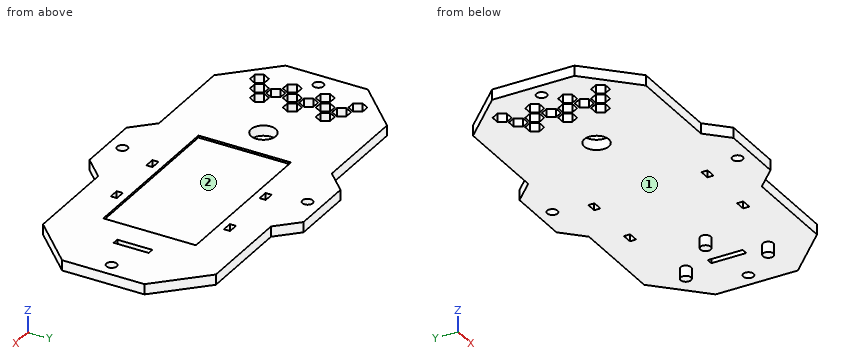
```python
from build123d import *

# Parameters (mm, degrees)
BASE_FLANGE1_OUTLINE_R  = 6
BASE_FLANGE1_DEPTH      = 5
SKETCH3_W               = 80
SKETCH3_H               = 45
CUT_EXTRUDE1_DEPTH      = 1
CROQUIS1_W              = 5
CROQUIS1_H              = 3
CORTAR_EXTRUIR1_DEPTH   = 108.540687679
CROQUIS2_R              = 2.5
CORTAR_EXTRUIR2_DEPTH   = 108.540687679
CROQUIS3_R              = 2.5
SALIENTE_EXTRUIR1_DEPTH = 5
CUT_EXTRUDE3_DEPTH      = 10
SKETCH9_W               = 3
SKETCH9_H               = 17
CUT_EXTRUDE4_DEPTH      = 10


# Read off the part's stored shape, not the designer's step: Base-Flange1
with BuildPart() as part:
    # Base-Flange1 outline → Base-Flange1 (new body)
    with BuildSketch(Plane(origin=(0, 0, 12.500000186), x_dir=(-1, 0, 0), z_dir=(0, 0, -1))):
        Polygon((-93.999996781, 19.999999553), (-93.999996781, -19.999999553), (-71.999996901, -41.999999434), (-25.556499138, -41.999999434), (-15.556500293, -52.000001073), (15.556500293, -52.000001073), (25.556499138, -41.999999434), (71.999996901, -41.999999434), (93.999996781, -19.999999553), (93.999996781, 19.999999553), (71.999996901, 41.999999434), (25.556499138, 41.999999434), (15.556500293, 52.000001073), (-15.556500293, 52.000001073), (-25.556499138, 41.999999434), (-71.999996901, 41.999999434), align=None)
        with Locations((40.791069868, 0)):
            Circle(BASE_FLANGE1_OUTLINE_R, mode=Mode.SUBTRACT)
    extrude(amount=BASE_FLANGE1_DEPTH)

    # Sketch3 → Cut-Extrude1 (cut)
    with BuildSketch(Plane.XY.offset(12.500000186)):
        with Locations((15, 0)):
            Rectangle(SKETCH3_W, SKETCH3_H)
    extrude(amount=-CUT_EXTRUDE1_DEPTH, mode=Mode.SUBTRACT)

    # Croquis1 → Cortar-Extruir1 (cut, through all)
    with BuildSketch(Plane.XY.offset(12.500000186)):
        with Locations((5, 27.5)):
            Rectangle(CROQUIS1_W, CROQUIS1_H)
        with Locations((35, 27.5)):
            Rectangle(CROQUIS1_W, CROQUIS1_H)
        with Locations((35, -27.5)):
            Rectangle(CROQUIS1_W, CROQUIS1_H)
        with Locations((5, -27.5)):
            Rectangle(CROQUIS1_W, CROQUIS1_H)
    extrude(amount=-CORTAR_EXTRUIR1_DEPTH, mode=Mode.SUBTRACT)

    # Croquis2 → Cortar-Extruir2 (cut, through all)
    with BuildSketch(Plane(origin=(0, 0, 7.500000186), x_dir=(-1, 0, 0), z_dir=(0, 0, -1))):
        with Locations((-86.999996781, 0)):
            Circle(CROQUIS2_R)
        with Locations(Location((86.999996781, 0, 0), (0, 0, 180))):
            Circle(CROQUIS2_R)
        with Locations((0, 45.000001073)):
            Circle(CROQUIS2_R)
        with Locations(Location((0, -45.000001073, 0), (0, 0, 180))):
            Circle(CROQUIS2_R)
    extrude(amount=-CORTAR_EXTRUIR2_DEPTH, mode=Mode.SUBTRACT)

    # Croquis3 → Saliente-Extruir1 (add)
    with BuildSketch(Plane(origin=(0, 0, 7.500000186), x_dir=(-1, 0, 0), z_dir=(0, 0, -1))):
        with Locations((-50.999996781, 0)):
            Circle(CROQUIS3_R)
        with Locations((-68.999996781, 20)):
            Circle(CROQUIS3_R)
        with Locations((-68.999996781, -20)):
            Circle(CROQUIS3_R)
    extrude(amount=SALIENTE_EXTRUIR1_DEPTH)

    # Sketch8 → Cut-Extrude3 (cut)
    with BuildSketch(Plane.XY.offset(12.500000186)):
        Polygon((-67.999996901, -19.999999553), (-69.999996901, -16.535897938), (-73.999996901, -16.535897938), (-75.999996901, -19.999999553), (-73.999996901, -23.464101168), (-69.999996901, -23.464101168), align=None)
        Polygon((-69.999996901, -8.607694708), (-67.999996901, -12.071796323), (-69.999996901, -15.535897938), (-73.999996901, -15.535897938), (-75.999996901, -12.071796323), (-73.999996901, -8.607694708), align=None)
        Polygon((-63.133971497, -19.499999553), (-67.133971497, -19.499999553), (-69.133971497, -16.035897938), (-67.133971497, -12.571796323), (-63.133971497, -12.571796323), (-61.133971497, -16.035897938), align=None)
        Polygon((-67.999996901, -3.999999553), (-69.999996901, -0.535897938), (-73.999996901, -0.535897938), (-75.999996901, -3.999999553), (-73.999996901, -7.464101168), (-69.999996901, -7.464101168), align=None)
        Polygon((-76.866022304, -27.428202783), (-80.866022304, -27.428202783), (-82.866022304, -23.964101168), (-80.866022304, -20.499999553), (-76.866022304, -20.499999553), (-74.866022304, -23.964101168), align=None)
        Polygon((-69.999996901, 7.392305292), (-67.999996901, 3.928203677), (-69.999996901, 0.464102062), (-73.999996901, 0.464102062), (-75.999996901, 3.928203677), (-73.999996901, 7.392305292), align=None)
        Polygon((-63.133971497, -3.499999553), (-67.133971497, -3.499999553), (-69.133971497, -0.035897938), (-67.133971497, 3.428203677), (-63.133971497, 3.428203677), (-61.133971497, -0.035897938), align=None)
        Polygon((-76.866022304, -11.428202783), (-80.866022304, -11.428202783), (-82.866022304, -7.964101168), (-80.866022304, -4.499999553), (-76.866022304, -4.499999553), (-74.866022304, -7.964101168), align=None)
        Polygon((-67.999996901, 12.000000447), (-69.999996901, 15.464102062), (-73.999996901, 15.464102062), (-75.999996901, 12.000000447), (-73.999996901, 8.535898832), (-69.999996901, 8.535898832), align=None)
        Polygon((-69.999996901, 23.392305292), (-67.999996901, 19.928203677), (-69.999996901, 16.464102062), (-73.999996901, 16.464102062), (-75.999996901, 19.928203677), (-73.999996901, 23.392305292), align=None)
        Polygon((-63.133971497, 12.500000447), (-67.133971497, 12.500000447), (-69.133971497, 15.964102062), (-67.133971497, 19.428203677), (-63.133971497, 19.428203677), (-61.133971497, 15.964102062), align=None)
        Polygon((-76.866022304, 4.571797217), (-80.866022304, 4.571797217), (-82.866022304, 8.035898832), (-80.866022304, 11.500000447), (-76.866022304, 11.500000447), (-74.866022304, 8.035898832), align=None)
        Polygon((-74.866022304, 23.892305292), (-76.866022304, 27.356406908), (-80.866022304, 27.356406908), (-82.866022304, 23.892305292), (-80.866022304, 20.428203677), (-76.866022304, 20.428203677), align=None)
    extrude(amount=-CUT_EXTRUDE3_DEPTH, mode=Mode.SUBTRACT)

    # Sketch9 → Cut-Extrude4 (cut)
    with BuildSketch(Plane.XY.offset(12.500000186)):
        with Locations((68.999996781, 0)):
            Rectangle(SKETCH9_W, SKETCH9_H)
    extrude(amount=-CUT_EXTRUDE4_DEPTH, mode=Mode.SUBTRACT)


solid = part.part
```
Here's how the part is built. I have some questions about the finished solid (model axes, mm). Face numbers are marked on the shaded views. Give positions to 0.01 mm unless a question says otherwise; leave off trailing zeros. Loops run counter-clockwise (first coordinate to the right, second up) from the corner with the lowest first, then second, coordinate; pieces in that order, holes last. Notation, with made-up numbers: M 58.5,86 L 64.5,86 A25 ccw 64.5,102 Z; hole C -14,47.25 d10. An arc over 180 degrees is marked long. Use one line per item in the form item = value. Start each with the question number.
Q1. If we section it at A-A (x = 0): Write out the boundary of the cut face in (y, z).
Q2. If we section it at B-B (x = 42): Write out the boundary of the cut face in (y, z), then the cut area to 3 significant figures.
Q3. If we section it at D-D (y = -33.5): Write out the boundary of the cut face in (x, z).
Q4. I need wall thicknesses on line 1 along Y through (x, z) = (35.5, 11.75); line 2 along Y through (x, z) = (0, 10.15); line 3 along Z through (x, y) = (66.5, 16.5). Which ranges of each line are inside material? Lowest first, please.
Q5. Thinking about a two-plate mould opening in X: for the marked faces 1 and 2, which applies, +X half, -X half, draft (parallel to the pull), parting line (faces both ways), or undercut?
Q6. If we section it at C-C (z = 4.5): Write out the boundary of the cut face in (x, y), then the cut area to 3 significant figures.
Q7. Will these pins go through, and if not, where does the flat tip stop? pin 1 Ø10 at (x, y) = (15.5, 10.5) entering from +Z; pin 2 Ø3 at (x, z) = (-72, 9.5) entering from +Y; pin 3 Ø3 at (x, z) = (-72, 9.5) entering from -Y; pin 4 Ø4 at (x, y) = (-87, 0) entering from +Z.
Taken from the geometry:
q1.outline = M -52,7.5 L -47.5,7.5 L -47.5,12.5 L -52,12.5 Z; M -42.5,7.5 L 42.5,7.5 L 42.5,12.5 L 22.5,12.5 L 22.5,11.5 L -22.5,11.5 L -22.5,12.5 L -42.5,12.5 Z; M 47.5,7.5 L 52,7.5 L 52,12.5 L 47.5,12.5 Z
q2.outline = M -42,7.5 L 42,7.5 L 42,12.5 L 22.5,12.5 L 22.5,11.5 L -22.5,11.5 L -22.5,12.5 L -42,12.5 Z
q2.area = 375 mm^2
q3.outline = M -80.5,7.5 L 80.5,7.5 L 80.5,12.5 L -80.5,12.5 Z
q4.line_1 = -42 to -29, -26 to -22.5, 22.5 to 26, 29 to 42
q4.line_2 = -52 to -47.5, -42.5 to 42.5, 47.5 to 52
q4.line_3 = 7.5 to 12.5
q5.face_1 = draft
q5.face_2 = undercut
q6.outline = C 51,0 d5; C 69,-20 d5; C 69,20 d5
q6.area = 58.9 mm^2
q7.pin_1 = 11.5
q7.pin_2 = 42
q7.pin_3 = -42
q7.pin_4 = through
